Answer from the drawing. Dimensions are ordinates in mm from the lowest x, y and z of the part. A direction names the side the tool comes from. Give positions to 0.01 mm unless a question says otherwise; leave off trailing zeros. Loops run counter-clockwise (first coordinate to the right, second up) from the corner with the lowest first, then second, coordinate; pieces in that order, holes last.
Item 1: Section B-B, the plane z = 10 is taken. Give the vertices of the cut face in (x, y), and give its area (3 significant figures).
Item 2: Section D-D, the plane z = 16.75 is taken. Give the vertices of the cut face in (x, y), and give its area (3 significant figures).
Item 3: Section A-A, the plane x = 10 is taken. Give the vertices of the cut face in (y, z).
Item 4: A tool of negligible diameter and unlimited length cuts with its end or side. For the marked faces 1 and 2, from which of +Z, -Z, +X, -X, +Y, -Y can it reach the whole face along a straight path? Write none if from no direction.
Item 5: Section C-C, the plane y = 2.3 is taken. Give the vertices of the cut face in (x, z), and give its area (3 significant figures).
Item 6: The mould has two halves that part along Z. Classify the marked faces 3, 4 and 5: pulls with the +Z half, pulls with the -Z half, needs draft (parallel to the pull), parting line crosses it, or undercut.
Item 7: Each of these flat-tipped pins is pushed along its axis until it touches: pin 1 Ø8 at (x, z) = (13, 3.5) entering from -Y; pin 2 Ø1.6 at (x, y) = (10, 3) entering from -Z. Where does it stop, or does it pass through?
Item 8: Consider line 1 along X through (y, z) = (1.2, 10); line 2 along Y through (x, z) = (16.75, 15.75); line 3 along Z through (x, y) = (7.5, 0.6). Determine where each line is inside the solid, lowest interval first.
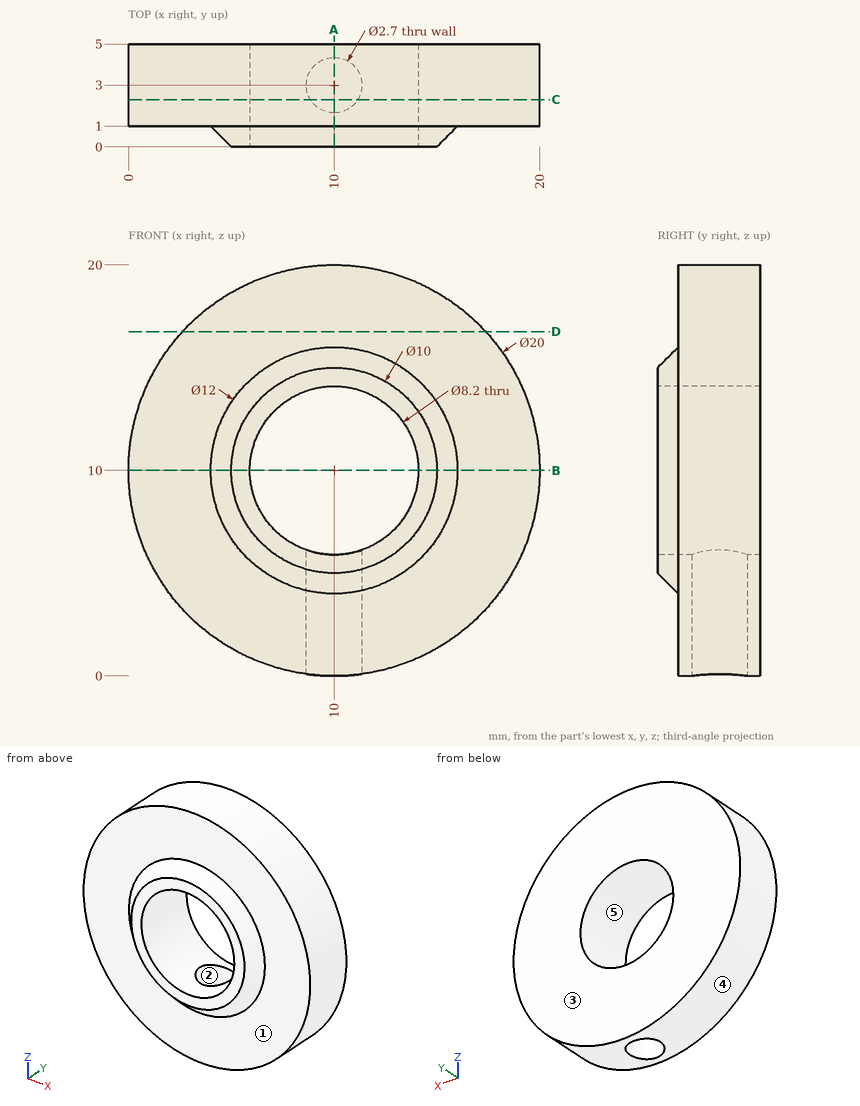
Worked answers:
1. outline: (0, 1) - (4, 1) - (5, 0) - (5.9, 0) - (5.9, 5) - (0, 5) - close; (14.1, 0) - (15, 0) - (16, 1) - (20, 1) - (20, 5) - (14.1, 5) - close
1. area: 50.0 mm2
2. outline: (2.62, 1) - (17.38, 1) - (17.38, 5) - (2.62, 5) - close
2. area: 59.0 mm2
3. outline: (0, 5) - (1, 4) - (1, 0) - (1.65, 0) - (1.65, 5.9) - (0, 5.9) - close; (0, 14.1) - (5, 14.1) - (5, 20) - (1, 20) - (1, 16) - (0, 15) - close; (4.35, 0) - (5, 0) - (5, 5.9) - (4.35, 5.9) - close
4. face 1: -Y
4. face 2: -Z
5. outline: (8.85, 0.07) - (8.85, 6.07) arc R4.1 cw (long way) to (11.15, 6.07) - (11.15, 0.07) arc R10 ccw (long way) to start
5. area: 248 mm2
6. face 3: needs draft
6. face 4: parting line crosses it
6. face 5: undercut
7. pin 1: stops at y = 0
7. pin 2: stops at z = 14.02
8. line 1: x = 0 to 5.9, 14.1 to 20
8. line 2: y = 1 to 5
8. line 3: z = 4.99 to 6.75, 13.25 to 15.01
